```python
from build123d import *

# Parameters (mm, degrees)
BOX001_W      = 5
BOX001_H      = 5
BOX001_DEPTH  = 5
ARRAY_X_COUNT = 5
ARRAY_X_PITCH = 10
ARRAY_Y_COUNT = 5
ARRAY_Y_PITCH = 10
BOX_W         = 50
BOX_H         = 50
BOX_DEPTH     = 5


with BuildPart() as array:
    # Box001 → Box001 (new body)
    with BuildSketch(Plane.XY):
        with Locations((2.5, 2.5)):
            Rectangle(BOX001_W, BOX001_H)
    extrude(amount=BOX001_DEPTH)

    # Array X: Array ×5


with BuildPart() as array_1:
    add(array.part)
    with Locations(*[(i * ARRAY_X_PITCH, 0, 0) for i in range(1, ARRAY_X_COUNT)]):
        add(array.part)

    # Array Y: Array ×5


with BuildPart() as array_2:
    add(array_1.part)
    with Locations(*[(0, i * ARRAY_Y_PITCH, 0) for i in range(1, ARRAY_Y_COUNT)]):
        add(array_1.part)


with BuildPart() as array_3:
    # Array placement: moved
    add(array_2.part.moved(Location((2.5, 2.5, 0))))


with BuildPart() as cut:
    # Box → Box (new body)
    with BuildSketch(Plane.XY):
        with Locations((25, 25)):
            Rectangle(BOX_W, BOX_H)
    extrude(amount=BOX_DEPTH)

    # Cut: cut Array
    add(array_3.part, mode=Mode.SUBTRACT)


solid = cut.part
```
Could you check a few things on this model? Use its own coordinates, in mm. Coordinates: 2 decimals unless noted, no trailing zeros. Write each loop counter-clockwise with the first axis right and the second up, starting at its lowest first coordinate (ties: lowest second). Pieces come first, ordered by that corner, then holes. Notation, with made-up numbers: (5.5, 23) -> (46.5, 23) arc R22 cw to (46.5, 60) -> close; hole circle Ø4 at (84.25, -13.75). An arc over 180 degrees is marked (long way). Write item = value, one per line. Start each with the question number.
(1) We'd pull the mould along Y, two halves only. Please class faces 1 (the face through (19, 25, 5)), 2 (the face through (25, 50, 2)), 3 (the face through (47.5, 45, 2)): released by +Y, released by -Y, zero draft, split by the parting line, or undercut.
(2) I want a section at A-A (y = 34.5). Please give me the cut outline in (x, z).
(3) I want a section at C-C (z = 4.25). Give the number of separate pieces and of enclosed holes in the cut face, plus the area to 4 significant figures.
(4) I need wall thicknesses on line 1 (Y direction, x = 23.5, z = 0.7). Which ranges of the line are inside material? Lowest first, please. Write a range as [from, to].
Result set:
q1.face_1 = zero draft
q1.face_2 = released by +Y
q1.face_3 = undercut
q2.outline = (0, 0) -> (2.5, 0) -> (2.5, 5) -> (0, 5) -> close; (7.5, 0) -> (12.5, 0) -> (12.5, 5) -> (7.5, 5) -> close; (17.5, 0) -> (22.5, 0) -> (22.5, 5) -> (17.5, 5) -> close; (27.5, 0) -> (32.5, 0) -> (32.5, 5) -> (27.5, 5) -> close; (37.5, 0) -> (42.5, 0) -> (42.5, 5) -> (37.5, 5) -> close; (47.5, 0) -> (50, 0) -> (50, 5) -> (47.5, 5) -> close
q3.separate_pieces = 1
q3.enclosed_holes = 25
q3.area = 1,875 mm2
q4.line_1 = [0, 2.5], [7.5, 12.5], [17.5, 22.5], [27.5, 32.5], [37.5, 42.5], [47.5, 50]
